Part model, mm, in its own coordinate system. Face numbers are marked on the shaded views. A direction names the side the tool comes from. Round coordinates to 2 decimals unless told otherwise and drop trailing zeros. Write each loop counter-clockwise with the first axis right and the second up, starting at its lowest first coordinate (ties: lowest second). Pieces come first, ordered by that corner, then holes. Notation, with made-up numbers: M 11.5,88 L 46.5,88 A8 cw 46.5,102 Z; hole C 0,84 d11. An arc over 180 degrees is marked long. One line per question, with ' | ' between items. Start each with the question number.
1) Drop flat-ended pins along their axis: pin 1 Ø2.5 at (x, y) = (12.7, 6.35) entering from -Z; pin 2 Ø2 at (x, y) = (8.5, 4) entering from +Z; pin 3 Ø4 at (y, z) = (6, 7.5) entering from -X. Give the stop position or say it passes through.
2) Saw through at D-D (y = 5.75). List the corners of the cut face in (x, z), plus the area to 3 significant figures.
3) Tool access for the marked faces 4 and 5: list every direction of +Z, -Z, +X, -X, +Y, -Y with a clear straight run to the whole face (end or side of a thin tool).
4) Saw through at A-A (x = 5.08). List the corners of the cut face in (y, z).
5) Saw through at B-B (y = 4.25). List the corners of the cut face in (x, z), plus the area to 3 significant figures.
6) Mould opens along Z. For the marked faces 1, 2 and 3 say: pulls with the +Z half, pulls with the -Z half, needs draft (parallel to the pull), parting line crosses it, or undercut.
7) Wall check: probe 1 along Z at (x, y) = (17.25, 6.35); probe 2 along Z at (x, y) = (17.25, 11.5); probe 3 along X at (y, z) = (12, 29.5). Give the ranges that are in metal, low to high. Write a range as [from, to].
8) Saw through at C-C (z = 11). List the corners of the cut face in (x, y), plus the area to 3 significant figures.
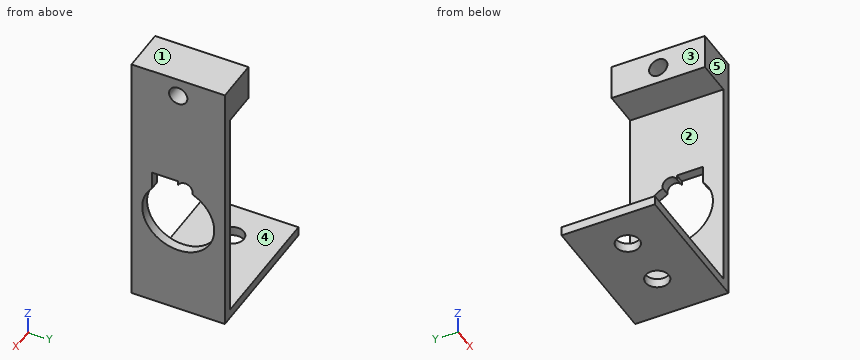
Autodesk Inventor part; units mm, degrees
ref_plane "YZ Plane" through (0, 0, 0) normal (1, 0, 0) x (0, 1, 0)
ref_plane "XZ Plane" through (0, 0, 0) normal (0, 1, 0) x (-1, 0, 0)
ref_plane "XY Plane" through (0, 0, 0) normal (0, 0, 1) x (1, 0, 0)
sketch "Sketch1" plane through (0, 0, 0) normal (0, 0, 1) x (1, 0, 0)
  line L0 (0, 0) -> (19.05, 0)
  line L1 (19.05, 0) -> (19.05, 12.7)
  line L2 (19.05, 12.7) -> (0, 12.7)
  line L3 (0, 12.7) -> (0, 0)
  circle A0 centre (5.08, 6.35) radius 1.5875
  circle A1 centre (12.7, 6.35) radius 1.5875
  dimension "d0" = 12.7
  dimension "d1" = 19.05
  dimension "d2" = 3.175
  dimension "d3" = 3.175
  dimension "d4" = 6.35
  dimension "d5" = 5.08
  dimension "d6" = 7.62
extrude "Extrusion1" add sketch "Sketch1" along normal blind 1.27
sketch "Sketch2" plane through (0, 0, 1.27) normal (0, 0, 1) x (1, 0, 0)
  line L0 (19.05, 12.7) -> (0, 12.7)
  line L1 (19.05, 0) -> (17.78, 0)
  line L2 (17.78, 0) -> (17.78, 12.7)
  line L3 (17.78, 12.7) -> (19.05, 12.7)
  line L4 (19.05, 12.7) -> (19.05, 0)
  point P0 (0, 0)
  dimension "d9" = 1.27
extrude "Extrusion2" add sketch "Sketch2" along normal blind 34.29
sketch "Sketch3" plane through (17.78, 0, 1.27) normal (-1, 0, 0) x (0, 0, 1)
  line L0 (0, 12.7) -> (0, 0)
  line L1 (0, 12.7) -> (34.29, 12.7)
  arc A0 (17.2142, 8.2614) -> (16.0744, 2.794) centre (12.7, 6.35) ccw
  line L2 (17.6022, 6.35) -> (18.5128, 6.35)
  line L3 (18.5128, 6.35) -> (18.5128, 2.794)
  line L4 (18.5128, 2.794) -> (16.0744, 2.794)
  line L5 (16.0744, 2.794) -> (16.0744, 6.35)
  arc A1 (17.8973, 6.35) -> (17.2142, 8.2614) centre (17.5113, 7.2898) ccw
  point P0 (-1.27, 0)
  point P1 (17.2936, 6.35)
  dimension "d21" = 9.8044
  dimension "d22" = 12.7
  dimension "d23" = 6.35
  dimension "d24" = 3.556
  dimension "d25" = 2.4384
  dimension "d26" = 2.032
  dimension "d27" = 0.9398
  dimension "d28" = 3.556
extrude "Extrusion3" cut sketch "Sketch3" against normal blind 25.4
sketch "Sketch4" plane through (17.78, 0, 1.27) normal (-1, 0, 0) x (0, 0, 1)
  line L0 (34.29, 12.7) -> (29.464, 12.7)
  line L1 (29.464, 12.7) -> (29.464, 0)
  line L2 (29.464, 0) -> (34.29, 0)
  line L3 (34.29, 0) -> (34.29, 12.7)
  arc A0 (17.2142, 8.2614) -> (16.0744, 2.794) centre (12.7, 6.35) ccw
  line L4 (0, 0) -> (34.29, 0)
  point P0 (-1.27, 0)
  point P1 (31.877, 0)
  dimension "d29" = 16.764
extrude "Extrusion4" add sketch "Sketch4" along normal blind 4.826
sketch "Sketch5" plane through (12.954, 0, 1.27) normal (-1, 0, 0) x (0, 0, 1)
  line L0 (34.29, 12.7) -> (29.464, 12.7)
  line L1 (29.464, 12.7) -> (29.464, 0)
  line L2 (29.464, 0) -> (34.29, 0)
  line L3 (34.29, 0) -> (34.29, 12.7)
  point P0 (-1.27, 0)
  point P1 (31.8008, 6.35)
  dimension "d33" = 4.826
  dimension "d35" = 12.7
  dimension "d38" = 6.35
  dimension "d46" = 2.3368
hole "Hole1" at (12.954, 6.35, 33.0708) direction (1, 0, 0) diameter 2.4892 end through all
properties part number "000208"
Answer key:
1) pin 1: stops at z = 30.73 | pin 2: stops at z = 1.27 | pin 3: stops at x = 17.78
2) outline: M 0,0 L 3.61,0 L 3.61,1.27 L 0,1.27 Z; M 6.55,0 L 11.23,0 L 11.23,1.27 L 6.55,1.27 Z; M 12.95,30.73 L 17.78,30.73 L 17.78,19.78 L 19.05,19.78 L 19.05,31.98 L 12.95,31.98 Z; M 12.95,34.16 L 19.05,34.16 L 19.05,35.56 L 12.95,35.56 Z; M 14.17,0 L 19.05,0 L 19.05,9.1 L 17.78,9.1 L 17.78,1.27 L 14.17,1.27 Z | area: 56.7 mm2
3) face 4: -X, +Y, -Y | face 5: +Z, -Z, +X, -X, -Y
4) outline: M 0,0 L 4.76,0 L 4.76,1.27 L 0,1.27 Z; M 7.94,0 L 12.7,0 L 12.7,1.27 L 7.94,1.27 Z
5) outline: M 0,0 L 19.05,0 L 19.05,9.54 L 17.78,9.54 L 17.78,1.27 L 0,1.27 Z; M 12.95,30.73 L 17.78,30.73 L 17.78,19.78 L 19.05,19.78 L 19.05,35.56 L 12.95,35.56 Z | area: 78.0 mm2
6) face 1: pulls with the +Z half | face 2: undercut | face 3: needs draft
7) probe 1: z = [0, 1.27], [30.73, 31.83], [34.32, 35.56] | probe 2: z = [0, 1.27], [30.73, 35.56] | probe 3: x = [17.78, 19.05]
8) outline: M 17.78,0 L 19.05,0 L 19.05,2.45 L 17.78,2.45 Z; M 17.78,10.25 L 19.05,10.25 L 19.05,12.7 L 17.78,12.7 Z | area: 6.22 mm2
